For this review, use the dimensioned drawing (mm, ordinates from the lowest corner) and the shaded views. A direction names the side the tool comes from. Give positions to 0.01 mm unless a question says otherwise; leave off trailing zeros. Write each loop counter-clockwise with the first axis right and the second up, starting at its lowest first coordinate (ties: lowest second). Pieces come first, ordered by that corner, then holes. Notation, with made-up numbers: (-29, 37.5) -> (24, 37.5) arc R25 cw to (24, 50.5) -> close; hole circle Ø11 at (-19.75, 61). An arc over 180 degrees is marked (long way). Answer as CSV lines item,"result".
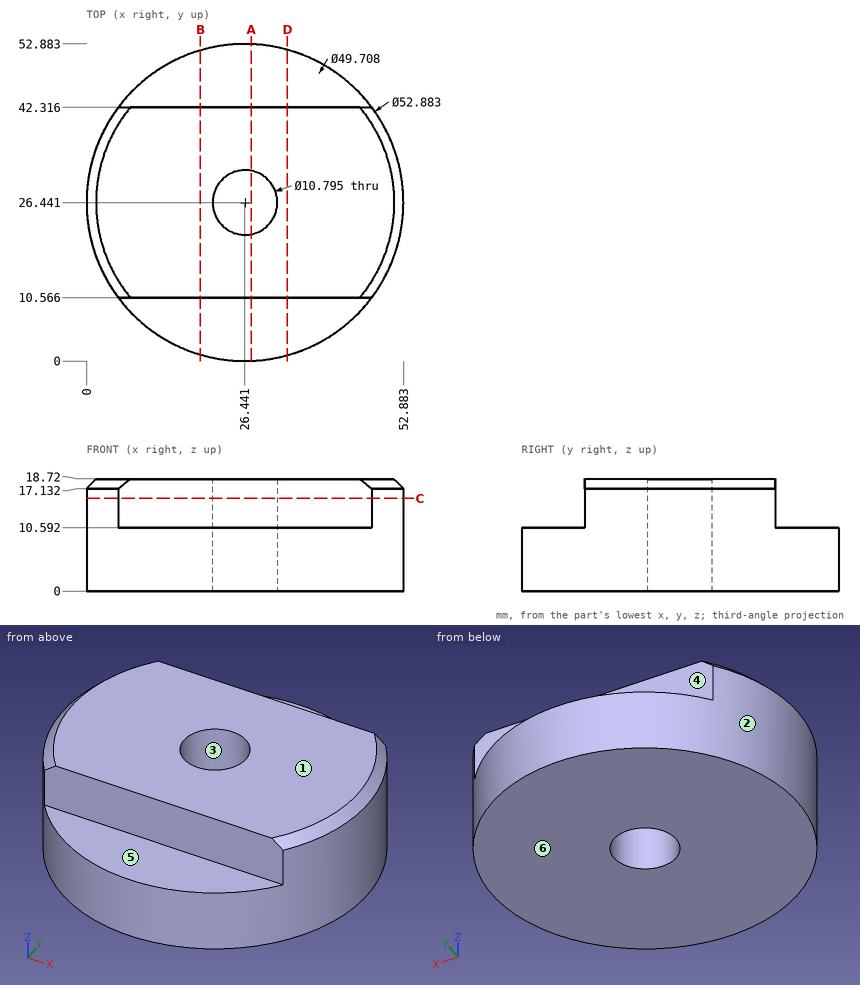
Q1. Draft analysis for pull direction X (two halves, no side actions). For the marked faces 1, 2 and 3, state which applies: released by +X, released by -X, zero draft, split by the parting line, or undercut.
Answer block:
face 1,"zero draft"
face 2,"split by the parting line"
face 3,"undercut"
Q2. To check wall thickness, follow probe 1 along Y at (x, z) = (33.5, 16.25); probe 2 along Y at (x, z) = (22, 11) (1 decimal); probe 3 along Z at (x, y) = (26, 50). State the ranges of each line that lie inside material, in increasing order. Write a range as [from, to].
Answer block:
probe 1,"y = [10.57, 42.32]"
probe 2,"y = [10.6, 23.4], [29.5, 42.3]"
probe 3,"z = [0, 10.59]"
Q3. For the marked faces 4, 5 and 6, list the 3-axis set-ups (+Z, -Z, +X, -X, +Y, -Y) from which the entire face can be reached by the end or side of a thin tool; tool diameter is ignored.
Answer block:
face 4,"+Z, +X, -X, +Y"
face 5,"+Z, +X, -X, -Y"
face 6,"-Z, +X, -X, +Y, -Y"
Q4. Add section A-A (x = 27.5). Write out the cut boundary in (y, z).
Answer block:
outline,"(0.02, 0) -> (21.15, 0) -> (21.15, 18.72) -> (10.57, 18.72) -> (10.57, 10.59) -> (0.02, 10.59) -> close; (31.73, 0) -> (52.86, 0) -> (52.86, 10.59) -> (42.32, 10.59) -> (42.32, 18.72) -> (31.73, 18.72) -> close"
Q5. Add section B-B (x = 19). Write out the cut boundary in (y, z).
Answer block:
outline,"(1.07, 0) -> (51.81, 0) -> (51.81, 10.59) -> (42.32, 10.59) -> (42.32, 18.72) -> (10.57, 18.72) -> (10.57, 10.59) -> (1.07, 10.59) -> close"
Q6. Add section D-D (x = 33.5). Write out the cut boundary in (y, z).
Answer block:
outline,"(0.96, 0) -> (51.92, 0) -> (51.92, 10.59) -> (42.32, 10.59) -> (42.32, 18.72) -> (10.57, 18.72) -> (10.57, 10.59) -> (0.96, 10.59) -> close"
Q7. Clearance check with flat-ended pins moving along their axes: pin 1 (4 mm diameter, centred on x = 18.5, z = 13.5, fed in from +Y); pin 2 (5 mm diameter, centred on y = 7, z = 2, fed in from -X); pin 3 (4 mm diameter, centred on x = 20.5, z = 8, fed in from +Y). State where each tip first meets the part, or that it passes through.
Answer block:
pin 1,"stops at y = 42.32"
pin 2,"stops at x = 6.14"
pin 3,"stops at y = 52.59"
Q8. Add section C-C (z = 15.5). Write out the cut boundary in (x, y) (1 decimal), plus the area to 3 significant figures.
Answer block:
outline,"(5.3, 10.6) -> (47.6, 10.6) arc R26.4 ccw to (47.6, 42.3) -> (5.3, 42.3) arc R26.4 ccw to start; hole circle Ø10.8 at (26.4, 26.4)"
area,"1,480 mm2"
